```python
from build123d import *

# Parameters (mm, degrees)
SKETCH_1_W          = 20
SKETCH_1_H          = 40.5
EXTRUDE_1_DEPTH     = 8.25
SKETCH_2_R          = 4
CUT_EXTRUDE_1_DEPTH = 17.5
SKETCH_3_R          = 6.5
CUT_EXTRUDE_2_DEPTH = 5
CHAMFER_1_SIZE      = 5
SKETCH_4_W          = 10
SKETCH_4_H          = 6
EXTRUDE_2_DEPTH     = 20
SKETCH_5_R          = 2.15
CUT_EXTRUDE_3_DEPTH = 17


with BuildPart() as part:
    # 草图1 → 凸台-拉伸1 (new body, symmetric)
    with BuildSketch(Plane.XY):
        with Locations((0, 20.25)):
            Rectangle(SKETCH_1_W, SKETCH_1_H)
    extrude(amount=EXTRUDE_1_DEPTH, both=True)

    # 草图2 → 切除-拉伸1 (cut, through all)
    with BuildSketch(Plane.XY.offset(8.25)):
        with Locations((0, 30.5)):
            Circle(SKETCH_2_R)
    extrude(amount=-CUT_EXTRUDE_1_DEPTH, mode=Mode.SUBTRACT)

    # 草图3 → 切除-拉伸2 (cut)
    with BuildSketch(Plane.XY.offset(8.25)):
        with Locations((0, 30.5)):
            Circle(SKETCH_3_R)
    cut_extrude_2 = extrude(amount=-CUT_EXTRUDE_2_DEPTH, mode=Mode.SUBTRACT)

    # 镜向1: 切除-拉伸2 across plane
    add(cut_extrude_2.mirror(Plane.XY), mode=Mode.SUBTRACT)

    # 倒角1
    chamfer_1_edges = [part.edges().sort_by_distance(p)[0] for p in [
        (-10, 40.5, 0),
        (10, 40.5, 0),
    ]]
    chamfer(chamfer_1_edges, length=CHAMFER_1_SIZE)

    # 草图4 → 凸台-拉伸2 (add)
    with BuildSketch(Plane(origin=(10, 0, 0), x_dir=(0, 0, -1), z_dir=(1, 0, 0))):
        with Locations((-13.25, 3)):
            Rectangle(SKETCH_4_W, SKETCH_4_H)
    extrude(amount=-EXTRUDE_2_DEPTH)

    # 草图5 → 切除-拉伸3 (cut)
    with BuildSketch(Plane(origin=(0, 6, 0), x_dir=(1, 0, 0), z_dir=(0, 1, 0))):
        with Locations((0, -14.25)):
            Circle(SKETCH_5_R)
    extrude(amount=-CUT_EXTRUDE_3_DEPTH, mode=Mode.SUBTRACT)


solid = part.part
```
Can you work these out from the model? Positions are in its coordinate system, mm. A direction names the side the tool comes from. Round coordinates to 2 decimals unless told otherwise and drop trailing zeros. Loops run counter-clockwise (first coordinate to the right, second up) from the corner with the lowest first, then second, coordinate; pieces in that order, holes last. Notation, with made-up numbers: M 36.25,-15 L 93.25,-15 A26 ccw 93.25,6 Z; hole C -2,25 d8. An arc over 180 degrees is marked long. Answer as a JSON object with one key per item and string values. Group by question number.
Q1. Imagine slicing it at A-A, the plane y = 30.5. Please give me the cut outline in (x, z), then the cut area to 3 significant figures.
Q2. Imagine slicing it at C-C, the plane z = 14.25. Please give me the cut outline in (x, y), then the cut area to 3 significant figures.
Q3. Will these pins go through, and if not, where does the flat tip stop? pin 1 (6 mm diameter, centred on x = 0.5, y = 23.5, fed in from +Z); pin 2 (10.5 mm diameter, centred on x = 0, y = 30.5, fed in from +Z).
Q4. Imagine slicing it at B-B, the plane x = 0. Please give me the cut outline in (y, z).
Q5. On a 3-axis mill with a long thin cutter (end or side, diameter ignored), from which of +Z, -Z, +X, -X, +Y, -Y can I reach the whole of each face in a straight line? I mean faces 1 (the flat face through (0, 26, 3.25)), 2 (the flat face through (0, 20, 8.25)), 3 (the cylindrical face through (-0.846, 36.945, -5.785)). Say none if no direction works.
Q6. We'd pull the mould along Y, two halves only. Please class faces 4 (the flat face through (0, 26, -3.25)), 5 (the flat face through (0, 3, 18.25)), 6 (the flat face through (0, 6, 11)): +Y half, -Y half, draft (parallel to the pull), parting line (faces both ways), or undercut.
Q7. Imagine slicing it at D-D, the plane z = 0.5. Please give me the cut outline in (x, y), then the cut area to 3 significant figures.
Q8. Please list where these lines run through material, in increasing order: L1, parallel to Z at x = 0, y = 3.85; L2, parallel to Y at x = 0, z = -6.45; L3, parallel to Z at x = 7, y = 28.
Findings:
{
 "1": {"outline": "M -10,-8.25 L -6.5,-8.25 L -6.5,-3.25 L -4,-3.25 L -4,3.25 L -6.5,3.25 L -6.5,8.25 L -10,8.25 Z; M 4,-3.25 L 6.5,-3.25 L 6.5,-8.25 L 10,-8.25 L 10,8.25 L 6.5,8.25 L 6.5,3.25 L 4,3.25 Z", "area": "148 mm2"},
 "2": {"outline": "M -10,0 L -2.15,0 L -2.15,6 L -10,6 Z; M 2.15,0 L 10,0 L 10,6 L 2.15,6 Z", "area": "94.2 mm2"},
 "3": {"pin 1": "stops at z = 8.25", "pin 2": "stops at z = 3.25"},
 "4": {"outline": "M 0,-8.25 L 24,-8.25 L 24,-3.25 L 26.5,-3.25 L 26.5,3.25 L 24,3.25 L 24,8.25 L 6,8.25 L 6,12.1 L 0,12.1 Z; M 0,16.4 L 6,16.4 L 6,18.25 L 0,18.25 Z; M 34.5,-3.25 L 37,-3.25 L 37,-8.25 L 40.5,-8.25 L 40.5,8.25 L 37,8.25 L 37,3.25 L 34.5,3.25 Z"},
 "5": {"face 1": "+Z", "face 2": "+Z, +X, -X, +Y", "face 3": "-Z"},
 "6": {"face 4": "undercut", "face 5": "draft", "face 6": "+Y half"},
 "7": {"outline": "M -10,0 L 10,0 L 10,35.5 L 5,40.5 L -5,40.5 L -10,35.5 Z; hole C 0,30.5 d8", "area": "735 mm2"},
 "8": {"L1": "z = -8.25 to 12.1, 16.4 to 18.25", "L2": "y = 0 to 24, 37 to 40.5", "L3": "z = -8.25 to 8.25"}
}
